from build123d import *

# Parameters (mm, degrees)
SKETCH_1_R          = 12.5
EXTRUDE_1_DEPTH     = 12
SKETCH_2_W          = 4
SKETCH_2_H          = 3.769678913
SKETCH_2_H_2        = 4
CUT_EXTRUDE_1_DEPTH = 22.365860619
SKETCH_3_R          = 6.5
CUT_EXTRUDE_2_DEPTH = 22.272047386
SKETCH_5_R          = 17.5
EXTRUDE_1_2_DEPTH   = 4
SKETCH_4_R          = 3
SKETCH_4_R_2        = 1.5
SKETCH_4_R_3        = 6.5
CUT_EXTRUDE_3_DEPTH = 30.470324057
FILLET_2_R          = 2


with BuildPart() as part:
    # 草图1 → Extrude 1 (new body)
    with BuildSketch(Plane.XY):
        Circle(SKETCH_1_R)
    extrude(amount=EXTRUDE_1_DEPTH)

    # 草图2 → 切除-拉伸1 (cut, through all)
    with BuildSketch(Plane.XY.offset(12)):
        with Locations((0, -12.384839456)):
            Rectangle(SKETCH_2_W, SKETCH_2_H)
        with Locations((0, 12.5)):
            Rectangle(SKETCH_2_W, SKETCH_2_H_2)
    extrude(amount=-CUT_EXTRUDE_1_DEPTH, mode=Mode.SUBTRACT)

    # 草图3 → 切除-拉伸2 (cut, through all)
    with BuildSketch(Plane.XY.offset(12)):
        Circle(SKETCH_3_R)
    extrude(amount=-CUT_EXTRUDE_2_DEPTH, mode=Mode.SUBTRACT)

    # 草图5 → Extrude 1 2 (add)
    with BuildSketch(Plane(origin=(0, 0, 12), x_dir=(-1, 0, 0), z_dir=(0, 0, -1))):
        Circle(SKETCH_5_R)
    extrude(amount=-EXTRUDE_1_2_DEPTH)

    # 草图4 → 切除-拉伸3 (cut, through all)
    with BuildSketch(Plane.XY.offset(16)):
        with Locations((8.838834765, 8.838834765)):
            Circle(SKETCH_4_R)
        with Locations((-8.838834765, 8.838834765)):
            Circle(SKETCH_4_R_2)
        with Locations(Location((-8.838834765, -8.838834765, 0), (0, 0, 321.892102579))):
            Circle(SKETCH_4_R)
        with Locations(Location((8.838834765, -8.838834765, 0), (0, 0, 48.439812768))):
            Circle(SKETCH_4_R_2)
        Circle(SKETCH_4_R_3)
    extrude(amount=-CUT_EXTRUDE_3_DEPTH, mode=Mode.SUBTRACT)

    # 圆角2
    fillet_2_edges = [part.edges().sort_by_distance(p)[0] for p in [
        (-2, -11.41948134, 12),
        (2, -11.41948134, 12),
        (2, 11.41948134, 12),
        (-2, 11.41948134, 12),
    ]]
    fillet(fillet_2_edges, radius=FILLET_2_R - 0.0001)  # a hair under: the kernel refuses the full size


solid = part.part
Work out the finished part from the listing and answer in its coordinate system (mm). A direction names the side the tool comes from. Round coordinates to 2 decimals unless told otherwise and drop trailing zeros. Loops run counter-clockwise (first coordinate to the right, second up) from the corner with the lowest first, then second, coordinate; pieces in that order, holes last. Notation, with made-up numbers: (47.25, 59) -> (66.25, 59) arc R5 ccw to (66.25, 68) -> close; hole circle Ø6 at (-27.5, -13). An arc over 180 degrees is marked (long way). Use one line per item in the form item = value.
(1) Straight lines are drawn through the part: line 1 (X direction, y = -9, z = 14.25); line 2 (Y direction, x = 8, z = 12.5); line 3 (Y direction, x = 0.5, z = 13). For each, find the intervals that lie inside material, in ascending order.
Answer list:
line_1 = -15.01 to -11.83, -5.84 to 7.35, 10.33 to 15.01
line_2 = -15.56 to -10.08, -7.6 to 5.96, 11.72 to 15.56
line_3 = -17.49 to -6.48, 6.48 to 17.49
(2) For a pull along Y with two mould halves and no side action, classify faces 1 (the cylindrical face through (8.19, 5.91, 9.89)), 2 (the flat face through (-2, 11, 5)), 3 (the flat face through (0, 10.5, 6)) as released by +Y, released by -Y, zero draft, split by the parting line, or undercut.
Answer list:
face_1 = undercut
face_2 = zero draft
face_3 = released by +Y
(3) Find section D-D on x = 8.5. Give the vertices of the cut face in (y, z).
Answer list:
outline = (-15.3, 12) -> (-10.3, 12) -> (-10.3, 16) -> (-15.3, 16) -> close; (-7.38, 0) -> (5.86, 0) -> (5.86, 16) -> (-7.38, 16) -> close; (11.82, 12) -> (15.3, 12) -> (15.3, 16) -> (11.82, 16) -> close
(4) Find section C-C on z = 4.25. Give the vertices of the cut face in (x, y).
Answer list:
outline = (-10.69, -6.48) arc R3 cw to (-6.48, -10.69) arc R12.5 ccw to (-2, -12.34) -> (-2, -10.5) -> (2, -10.5) -> (2, -12.34) arc R12.5 ccw to (7.72, -9.83) arc R1.5 cw to (9.83, -7.72) arc R12.5 ccw to (10.69, 6.48) arc R3 cw to (6.48, 10.69) arc R12.5 ccw to (2, 12.34) -> (2, 10.5) -> (-2, 10.5) -> (-2, 12.34) arc R12.5 ccw to (-7.72, 9.83) arc R1.5 cw to (-9.83, 7.72) arc R12.5 ccw to start; hole circle Ø13 at (0, 0)
(5) Find section A-A on y = 0. Give the vertices of the cut face in (x, z).
Answer list:
outline = (-17.5, 12) -> (-12.5, 12) -> (-12.5, 0) -> (-6.5, 0) -> (-6.5, 16) -> (-17.5, 16) -> close; (6.5, 0) -> (12.5, 0) -> (12.5, 12) -> (17.5, 12) -> (17.5, 16) -> (6.5, 16) -> close
(6) A tool of negligible diameter and unlimited length cuts with its end or side. For faces 4 (the cylindrical face through (4.9, -11.5, 5.9)), 5 (the flat face through (5, -12, 12)), 6 (the flat face through (2, -11, 5)), 7 (the flat face through (2, 11, 5)), from which of +Z, -Z, +X, -X, +Y, -Y can it reach the whole face along a straight path? Write none if from no direction.
Answer list:
face_4 = -Z, +X, -Y
face_5 = -Z
face_6 = -Z, -Y
face_7 = -Z, +Y
(7) Find section B-B on x = 1. Give the vertices of the cut face in (y, z), then the cut area to 3 significant figures.
Answer list:
outline = (-17.47, 12) -> (-12.46, 12) -> (-12.46, 11.73) -> (-10.5, 11.73) -> (-10.5, 0) -> (-6.42, 0) -> (-6.42, 16) -> (-17.47, 16) -> close; (6.42, 0) -> (10.5, 0) -> (10.5, 11.73) -> (12.46, 11.73) -> (12.46, 12) -> (17.47, 12) -> (17.47, 16) -> (6.42, 16) -> close
area = 187 mm2
(8) Flat-ended cylindrical pins translate along their axes: P1, Ø5, axis at y = 5.5, z = 5, coming from the +X side; P2, Ø2, axis at y = 11.5, z = 6, coming from the +X side; P3, Ø2, axis at x = -0.5, z = 5, coming from the +Y side. Find the tip coordinate at first contact, or state that the pin passes through.
Answer list:
P1 = 12.13
P2 = 6.48
P3 = 10.5
